Geometry: final body of the model. Coordinates: model frame, mm. A direction names the side the tool comes from. Give positions to 0.01 mm unless a question says otherwise; leave off trailing zeros. Loops run counter-clockwise (first coordinate to the right, second up) from the corner with the lowest first, then second, coordinate; pieces in that order, holes last. Notation, with made-up numbers: (51, -14) - (88, -14) arc R16 ccw to (88, 14) - close; hole circle Ø10 at (-25.5, 72). An arc over 180 degrees is marked (long way). Use one line per item in the form item = value.
```python
from build123d import *

# Parameters (mm, degrees)
EXTRUSION12_DEPTH             = 4.25
ENL_V_MAT_EXTRU_13_DEPTH      = 5.25
ESQUISSE35_R                  = 5
ESQUISSE35_R_2                = 4.25
ENL_V_MAT_EXTRU_14_DEPTH      = 5.25
ENL_V_MAT_EXTRU_14_DEPTH_BACK = 5.25
ESQUISSE36_R                  = 6.15
ENL_V_MAT_EXTRU_15_DEPTH      = 2


with BuildPart() as part:
    # Esquisse33 → Extrusion12 (new body, symmetric)
    with BuildSketch(Plane.XY):
        with BuildLine():
            Line((10.891822315, -37.854750679), (13.257957999, -41.725))
            ThreePointArc((13.257957999, -41.725), (5.786859841, -39.732024729), (0.301056866, -34.282692308))
            ThreePointArc((0.301056866, -34.282692308), (-0.743831674, -31.380582548), (-0.684284829, -28.296674752))
            Line((-0.684284829, -28.296674752), (4.898579806, -1.001956028))
            ThreePointArc((4.898579806, -1.001956028), (1.001956028, 4.898579806), (-4.898579806, 1.001956028))
            Line((-4.898579806, 1.001956028), (-6.301318246, -5.8560557))
            Line((-6.301318246, -5.8560557), (-10.805878352, -4.934692503))
            ThreePointArc((-10.805878352, -4.934692503), (-11.858094208, -4.349595341), (-12.383780945, -3.266474687))
            Line((-12.383780945, -3.266474687), (-15.191076253, 15.807989781))
            ThreePointArc((-15.191076253, 15.807989781), (-10.881496713, 23.724620088), (-2.079236513, 21.784072078))
            Line((-2.079236513, 21.784072078), (4.917258536, 13.630466886))
            ThreePointArc((4.917258536, 13.630466886), (11.878383999, 8.981113225), (20.241537521, 8.618593782))
            ThreePointArc((20.241537521, 8.618593782), (21.960728113, -1.313933303), (19.069494762, -10.970613909))
            ThreePointArc((19.069494762, -10.970613909), (15.992864342, -19.46838522), (16.010964353, -28.505942654))
            ThreePointArc((16.010964353, -28.505942654), (15.098768048, -34.082402323), (10.891822315, -37.854750679))
        make_face()
    extrude(amount=EXTRUSION12_DEPTH, both=True)

    # Esquisse34 → Enlèv. mat.-Extru.13 (cut, through all)
    with BuildSketch(Plane.XY):
        with BuildLine():
            Line((4.898579806, -1.001956028), (3.495841367, -7.859967757))
            Line((3.495841367, -7.859967757), (11.333569057, -9.463097402))
            Line((11.333569057, -9.463097402), (12.53591629, -3.584801635))
            ThreePointArc((12.53591629, -3.584801635), (14.679166999, -0.414448762), (18.436452125, 0.311822143))
            Line((18.436452125, 0.311822143), (21.996061624, -0.416260758))
            ThreePointArc((21.996061624, -0.416260758), (21.596547051, 4.193942712), (20.241537521, 8.618593782))
            ThreePointArc((20.241537521, 8.618593782), (11.878383999, 8.981113225), (4.917258536, 13.630466886))
            Line((4.917258536, 13.630466886), (-2.079236513, 21.784072078))
            ThreePointArc((-2.079236513, 21.784072078), (-10.881496713, 23.724620088), (-15.191076253, 15.807989781))
            Line((-15.191076253, 15.807989781), (-12.383780945, -3.266474687))
            ThreePointArc((-12.383780945, -3.266474687), (-11.858094208, -4.349595341), (-10.805878352, -4.934692503))
            Line((-10.805878352, -4.934692503), (-6.301318246, -5.8560557))
            Line((-6.301318246, -5.8560557), (-4.898579806, 1.001956028))
            ThreePointArc((-4.898579806, 1.001956028), (1.001956028, 4.898579806), (4.898579806, -1.001956028))
        make_face()
    extrude(amount=ENL_V_MAT_EXTRU_13_DEPTH, mode=Mode.SUBTRACT)

    # Esquisse35 → Enlèv. mat.-Extru.14 (cut, two sides)
    with BuildSketch(Plane.XY) as enl_v_mat_extru_14_sk:
        with Locations((-7.771007489, 16.900042681)):
            Circle(ESQUISSE35_R)
        with Locations((7.643300841, -30)):
            Circle(ESQUISSE35_R_2)
    extrude(amount=ENL_V_MAT_EXTRU_14_DEPTH, mode=Mode.SUBTRACT)
    extrude(enl_v_mat_extru_14_sk.sketch, amount=-ENL_V_MAT_EXTRU_14_DEPTH_BACK, mode=Mode.SUBTRACT)

    # Esquisse36 → Enlèv. mat.-Extru.15 (cut)
    with BuildSketch(Plane(origin=(0, 0, -4.25), x_dir=(-1, 0, 0), z_dir=(0, 0, -1))):
        with Locations((7.771007489, 16.900042681)):
            Circle(ESQUISSE36_R)
    extrude(amount=-ENL_V_MAT_EXTRU_15_DEPTH, mode=Mode.SUBTRACT)


solid = part.part
```
(1) Cut plane A-A (y = -30). Return the cut outline in (x, z).
Solution:
outline = (-0.86, -4.25) - (3.39, -4.25) - (3.39, 4.25) - (-0.86, 4.25) - close; (11.89, -4.25) - (16.14, -4.25) - (16.14, 4.25) - (11.89, 4.25) - close
(2) Cut plane B-B (x = -10). Return the cut outline in (y, z).
Solution:
outline = (-5.1, -4.25) - (11.17, -4.25) - (11.17, -2.25) - (12.42, -2.25) - (12.42, 0) - (-5.1, 0) - close; (21.38, -2.25) - (22.63, -2.25) - (22.63, -4.25) - (24.06, -4.25) - (24.06, 0) - (21.38, 0) - close
(3) Pin query (flat end, axial travel): P1, Ø1, axis at y = -14.5, z = 0.5, coming from the +X side; P2, Ø7.5, axis at x = -7.77, y = 16.9, coming from the +Z side; P3, Ø3, axis at y = 6.5, z = 1, coming from the +X side; P4, Ø13.5, axis at x = -5, y = 15, coming from the -Z side. Return the tip coordinate at first contact, or that it passes through.
Solution:
P1 = 17.58
P2 = through
P3 = 21.33
P4 = -4.25
(4) Access query for faces 1 (the face through (20.191, -0.047, 2.095)), 2 (the face through (11.926, -6.565, 2.095)), 3 (the face through (-7, 22, -2.25)). Directions: +Z, -Z, +X, -X, +Y, -Y. A direction counts if a zero-diameter tool reaches every point of the face in a straight line with its end or side. Return the directions, or none.
Solution:
face_1 = +Z, +X, +Y
face_2 = +Z, +Y
face_3 = -Z
(5) Material intervals for L1, parallel to Y at x = 11.5, z = -3.25; L2, parallel to Z at x = 5, y = 12; L3, parallel to Y at x = 12, z = -0.75, sorted ascending. Write a range as from..to.
Solution:
L1 = -41.62..-38.85, -37.57..-31.79, -28.21..9.11
L2 = -4.25..0
L3 = -41.67..-39.67, -37.3..8.94
(6) Pull-direction query (X, two-part tool) for faces 4 (the face through (12.058, -39.763, 0.059)), 5 (the face through (-3, 18.4, -1.1)), 6 (the face through (-0.737, -31.423, 0.059)); classes: released by +X, released by -X, zero draft, split by the parting line, or undercut.
Solution:
face_4 = released by +X
face_5 = undercut
face_6 = released by -X
(7) Cut plane D-D (z = -3). Give the number of separate pieces and of enclosed holes in the cut face, plus the area to 3 significant figures.
Solution:
separate_pieces = 1
enclosed_holes = 2
area = 1,000 mm2
